from build123d import *
from build123d.topology import SkipClean

# Parameters (mm, degrees)
SKETCH1_W               = 21.76
SKETCH1_H               = 66
SKETCH1_W_2             = 62.8
BOSS_EXTRUDE1_DEPTH     = 10
SKETCH1_5_W             = 62.8
SKETCH1_5_H             = 66
CUT_EXTRUDE1_DEPTH      = 5
SKETCH3_R               = 7.65
SKETCH3_R_2             = 5.75
CUT_EXTRUDE2_DEPTH      = 62
CUT_EXTRUDE3_DEPTH      = 84.797288739
CUT_EXTRUDE3_DEPTH_BACK = 84.797288739
SKETCH3_3_R             = 5.75
BOSS_EXTRUDE2_DEPTH     = 5
CUT_EXTRUDE4_DEPTH      = 72.560503073
SKETCH5_R               = 30
CUT_EXTRUDE5_DEPTH      = 72.560503073
BOSS_EXTRUDE3_START     = 50
SKETCH5_3_R             = 30
BOSS_EXTRUDE3_DEPTH     = 50


with BuildPart() as part:
    # Sketch1 → Boss-Extrude1 (new body)
    with BuildSketch(Plane(origin=(0, 0, 0), x_dir=(1, 0, 0), z_dir=(0, 1, 0))):
        with Locations((-42.28, 0)):
            Rectangle(SKETCH1_W, SKETCH1_H)
        Rectangle(SKETCH1_W_2, SKETCH1_H)
        with Locations((42.28, 0)):
            Rectangle(SKETCH1_W, SKETCH1_H)
    extrude(amount=BOSS_EXTRUDE1_DEPTH)

    # Sketch1<5> → Cut-Extrude1 (cut)
    with BuildSketch(Plane(origin=(0, 0, 0), x_dir=(1, 0, 0), z_dir=(0, 1, 0))):
        Rectangle(SKETCH1_5_W, SKETCH1_5_H)
    extrude(amount=CUT_EXTRUDE1_DEPTH, mode=Mode.SUBTRACT)

    # Sketch3 → Cut-Extrude2 (cut)
    # profile 1 of 4: a face of its own
    with BuildSketch(Plane.XY.offset(31)):
        with Locations((-42.25, -4.5)):
            Circle(SKETCH3_R)
        with Locations((-42.25, -4.5)):
            Circle(SKETCH3_R_2, mode=Mode.SUBTRACT)
    # profile 2 of 4: a face of its own
    with BuildSketch(Plane.XY.offset(31)):
        with Locations((-42.25, -4.5)):
            Circle(SKETCH3_R_2)
    # profile 3 of 4: a face of its own
    with BuildSketch(Plane.XY.offset(31)):
        with Locations((42.31, -4.5)):
            Circle(SKETCH3_R)
        with Locations((42.31, -4.5)):
            Circle(SKETCH3_R_2, mode=Mode.SUBTRACT)
    # profile 4 of 4: a face of its own
    with BuildSketch(Plane.XY.offset(31)):
        with Locations((42.31, -4.5)):
            Circle(SKETCH3_R_2)
    extrude(amount=-CUT_EXTRUDE2_DEPTH, mode=Mode.SUBTRACT)

    # Sketch3<3> → Cut-Extrude3 (cut, two sides: drawn at the far end of the back side and taken through both)
    with BuildSketch(Plane.XY.offset(31).offset(-CUT_EXTRUDE3_DEPTH_BACK)):
        with Locations((42.31, -4.5)):
            Circle(SKETCH3_3_R)
        with Locations((-42.25, -4.5)):
            Circle(SKETCH3_3_R)
    extrude(amount=CUT_EXTRUDE3_DEPTH + CUT_EXTRUDE3_DEPTH_BACK, mode=Mode.SUBTRACT)

    # Sketch4 → Boss-Extrude2 (add)
    with BuildSketch(Plane.XZ):
        with BuildLine():
            Line((-51.16, 33), (-47.16, 33))
            ThreePointArc((-47.16, 33), (-57.402640687, 37.242640687), (-53.16, 27))
            Line((-53.16, 27), (-53.16, 31))
            ThreePointArc((-53.16, 31), (-54.574213562, 34.414213562), (-51.16, 33))
        make_face()
        with BuildLine():
            ThreePointArc((-53.16, -27), (-57.402640687, -37.242640687), (-47.16, -33))
            Line((-47.16, -33), (-51.16, -33))
            ThreePointArc((-51.16, -33), (-54.574213562, -34.414213562), (-53.16, -31))
            Line((-53.16, -31), (-53.16, -27))
        make_face()
        with BuildLine():
            ThreePointArc((47.16, -33), (57.402640687, -37.242640687), (53.16, -27))
            Line((53.16, -27), (53.16, -31))
            ThreePointArc((53.16, -31), (54.574213562, -34.414213562), (51.16, -33))
            Line((51.16, -33), (47.16, -33))
        make_face()
        with BuildLine():
            ThreePointArc((53.16, 27), (57.402640687, 37.242640687), (47.16, 33))
            Line((47.16, 33), (51.16, 33))
            ThreePointArc((51.16, 33), (54.574213562, 34.414213562), (53.16, 31))
            Line((53.16, 31), (53.16, 27))
        make_face()
    extrude(amount=-BOSS_EXTRUDE2_DEPTH)

    # Sketch4<3> → Cut-Extrude4 (cut, through all)
    with SkipClean():  # the faces are left unmerged after this step: merging them gives an invalid solid
        with BuildSketch(Plane.XZ):
            with BuildLine():
                ThreePointArc((51.16, 33), (51.745786438, 31.585786438), (53.16, 31))
                Line((53.16, 31), (53.16, 33))
                Line((53.16, 33), (51.16, 33))
            make_face()
            with BuildLine():
                Line((53.16, 33), (53.16, 31))
                ThreePointArc((53.16, 31), (54.574213562, 31.585786438), (55.16, 33))
                ThreePointArc((55.16, 33), (53.16, 35), (51.16, 33))
                Line((51.16, 33), (53.16, 33))
            make_face()
            with BuildLine():
                ThreePointArc((55.16, -33), (54.574213562, -31.585786438), (53.16, -31))
                Line((53.16, -31), (53.16, -33))
                Line((53.16, -33), (51.16, -33))
                ThreePointArc((51.16, -33), (53.16, -35), (55.16, -33))
            make_face()
            with BuildLine():
                Line((53.16, -33), (53.16, -31))
                ThreePointArc((53.16, -31), (51.745786438, -31.585786438), (51.16, -33))
                Line((51.16, -33), (53.16, -33))
            make_face()
            with BuildLine():
                ThreePointArc((-53.16, -31), (-54.574213562, -34.414213562), (-51.16, -33))
                Line((-51.16, -33), (-53.16, -33))
                Line((-53.16, -33), (-53.16, -31))
            make_face()
            with BuildLine():
                Line((-53.16, -33), (-51.16, -33))
                ThreePointArc((-51.16, -33), (-51.745786438, -31.585786438), (-53.16, -31))
                Line((-53.16, -31), (-53.16, -33))
            make_face()
            with BuildLine():
                ThreePointArc((-53.16, 31), (-51.745786438, 31.585786438), (-51.16, 33))
                Line((-51.16, 33), (-53.16, 33))
                Line((-53.16, 33), (-53.16, 31))
            make_face()
            with BuildLine():
                Line((-53.16, 33), (-51.16, 33))
                ThreePointArc((-51.16, 33), (-54.574213562, 34.414213562), (-53.16, 31))
                Line((-53.16, 31), (-53.16, 33))
            make_face()
        extrude(amount=-CUT_EXTRUDE4_DEPTH, mode=Mode.SUBTRACT)

    # Sketch5 → Cut-Extrude5 (cut, through all)
    with SkipClean():  # the faces are left unmerged after this step: merging them gives an invalid solid
        with BuildSketch(Plane(origin=(0, 10, 0), x_dir=(1, 0, 0), z_dir=(0, 1, 0))):
            with Locations(Location((4.77, 0, 0), (0, 0, 270))):
                Circle(SKETCH5_R)
        extrude(amount=-CUT_EXTRUDE5_DEPTH, mode=Mode.SUBTRACT)

    # Sketch5<3> → Boss-Extrude3 (add)
    with SkipClean():  # the faces are left unmerged after this step: merging them gives an invalid solid
        with BuildSketch(Plane(origin=(0, 10, 0), x_dir=(1, 0, 0), z_dir=(0, 1, 0)).offset(BOSS_EXTRUDE3_START)):
            with BuildLine():
                Line((-9.61749457, -33), (19.15749457, -33))
                ThreePointArc((19.15749457, -33), (34.886024011, -19.723719166), (40.77, 0))
                ThreePointArc((40.77, 0), (34.886024011, 19.723719166), (19.15749457, 33))
                Line((19.15749457, 33), (-9.61749457, 33))
                ThreePointArc((-9.61749457, 33), (-31.23, 0), (-9.61749457, -33))
            make_face()
            with Locations(Location((4.77, 0, 0), (0, 0, 270))):
                Circle(SKETCH5_3_R, mode=Mode.SUBTRACT)
        extrude(amount=-BOSS_EXTRUDE3_DEPTH)


solid = part.part
Input: part model. Units: mm. Frame: model coordinates. A direction names the side the tool comes from. Coordinates: 2 decimals unless noted, no trailing zeros. Order: outer loops, then holes, each group sorted by start corner. A loop starts at its lowest first (then second) coordinate and runs counter-clockwise, first axis right, second up. Notation, with made-up numbers: M 45,86.5 L 81,86.5 A25 cw 81,100.5 Z; hole C 60,-39 d10. An arc over 180 degrees is marked long. Answer in a Markdown table with one row per item.
(1) Draft query along Y for faces 4 (the cylindrical face through (-42.15, 3.15, 0.43)), 5 (the flat face through (-42, 2, 31)), 6 (the flat face through (-55, 5, -36)). Return one class per face: pulls with the +Y half, pulls with the -Y half, needs draft (parallel to the pull), parting line crosses it, or undercut.
Numbers:
| item | result |
|---|---|
| face 4 | pulls with the -Y half |
| face 5 | needs draft |
| face 6 | pulls with the +Y half |
(2) Material intervals for line 1 (Z direction, x = -53, y = 1); line 2 (Z direction, x = 6, y = 19.5); line 3 (X direction, y = 14, z = 22.5), sorted ascending. Write a range as [from, to].
Numbers:
| item | result |
|---|---|
| line 1 | z = [-39, -34.99], [-31.01, 31.01], [34.99, 39] |
| line 2 | z = [-33, -29.97], [29.97, 33] |
| line 3 | x = [-23.33, -15.07], [24.61, 32.87] |
(3) Section query B-B, the plane y = 55.5. Output: boundary loops of the cut face in (x, z).
Numbers:
| item | result |
|---|---|
| outline | M -9.62,-33 L 19.16,-33 A36 ccw 19.16,33 L -9.62,33 A36 ccw Z; hole C 4.77,0 d60 |
(4) Access query for faces 1 (the cylindrical face through (42.41, 3.15, 0.43)), 2 (the flat face through (52, 0, -1)), 3 (the flat face through (31.4, 2, -23)). Directions: +Z, -Z, +X, -X, +Y, -Y. A direction counts if a zero-diameter tool reaches every point of the face in a straight line with its end or side. Return the directions, or none.
Numbers:
| item | result |
|---|---|
| face 1 | -Y |
| face 2 | +Z, -Z, +X, -X, -Y |
| face 3 | +Z, -Z, -Y |
(5) Section query A-A, the plane x = 4.77. Output: boundary loops of the cut face in (y, z), plus the area to 3 significant figures.
Numbers:
| item | result |
|---|---|
| outline | M 5,-33 L 60,-33 L 60,-30 L 5,-30 Z; M 5,30 L 60,30 L 60,33 L 5,33 Z |
| area | 330 mm^2 |
(6) Contact query for flat-ended pins moving along their axis: pin 1 Ø3 at (x, y) = (-16.5, 12) entering from +Z; pin 2 Ø5 at (x, y) = (35, 32) entering from -Z; pin 3 Ø4 at (y, z) = (2.5, 13) entering from +X. Output: stop coordinate, or through.
Numbers:
| item | result |
|---|---|
| pin 1 | stops at z = 30.09 |
| pin 2 | stops at z = -22.96 |
| pin 3 | stops at x = 53.16 |
